Can you work these out from the model? Positions are in its coordinate system, mm. Round coordinates to 2 decimals unless told otherwise and drop trailing zeros. Order: outer loops, then holes, each group sorted by start corner. A loop starts at its lowest first (then second) coordinate and runs counter-clockwise, first axis right, second up.
Q1. If we section it at C-C (y = 50): Please give me the cut outline in (x, z).
Q2. If we section it at B-B (x = 0): Please give me the cut outline in (y, z), plus the area to 3 significant figures.
Q3. Will these pins go through, and if not, where does the flat tip stop? P1, Ø0.5, axis at x = 39.5, z = 1, coming from the -Y side; P2, Ø0.8, axis at y = 0.5, z = 0.5, coming from the -X side; P3, Ø0.5, axis at x = 52, z = 0.5, coming from the +Y side; P4, Ø0.5, axis at x = -40.5, z = 0.5, coming from the -Y side.
Q4. If we section it at A-A (y = 0): Please give me the cut outline in (x, z) (3 decimals), plus the area to 3 significant figures.
Q5. If we section it at D-D (z = 0.3): Count the separate pieces of the cut face and the enclosed holes in it, plus the area to 3 significant figures.
Q6. If I drill on line 1 (Y direction, x = 0, z = 0.55); line 2 (Y direction, x = 18.5, z = 1.45); line 3 (X direction, y = 46, z = 0.3) (3 decimals), over which ranges is the centre line in solid material (lowest first)?
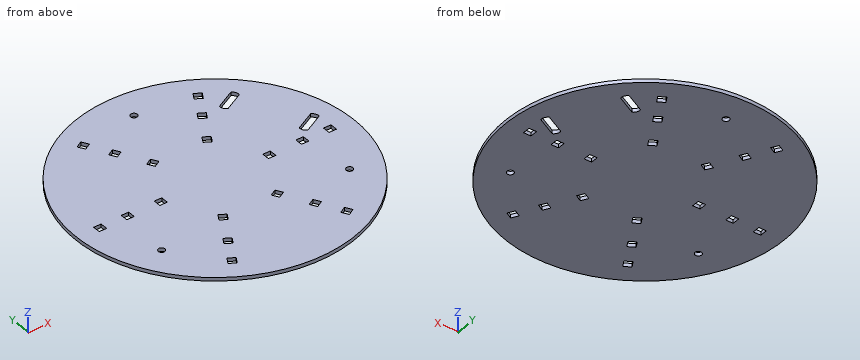
from build123d import *

# Parameters (mm, degrees)
SKETCH1_R           = 63.5
BOSS_EXTRUDE1_DEPTH = 1.6
SKETCH3_R           = 1.75
CUT_EXTRUDE4_DEPTH  = 1.6
SKETCH2_R           = 1.5
CUT_EXTRUDE5_DEPTH  = 1.6
CUT_EXTRUDE6_DEPTH  = 10
SKETCH5_W           = 3.45
SKETCH5_H           = 3.45
CUT_EXTRUDE7_DEPTH  = 10


with BuildPart() as part:
    # Sketch1 → Boss-Extrude1 (new body)
    with BuildSketch(Plane.XY):
        Circle(SKETCH1_R)
    extrude(amount=BOSS_EXTRUDE1_DEPTH)

    # Sketch3 → Cut-Extrude4 (cut)
    with BuildSketch(Plane(origin=(0, 0, 0), x_dir=(-1, 0, 0), z_dir=(0, 0, -1))):
        with Locations((-34.006305458, 36.654756705)):
            Circle(SKETCH3_R)
        with Locations((-49.354669589, 8.007283544)):
            Circle(SKETCH3_R)
    extrude(amount=-CUT_EXTRUDE4_DEPTH, mode=Mode.SUBTRACT)

    # Sketch2 → Cut-Extrude5 (cut)
    with BuildSketch(Plane(origin=(0, 0, 0), x_dir=(-1, 0, 0), z_dir=(0, 0, -1))):
        with Locations((0, 50)):
            Circle(SKETCH2_R)
        with Locations((43.301270189, -25)):
            Circle(SKETCH2_R)
        with Locations((-43.301270189, -25)):
            Circle(SKETCH2_R)
    extrude(amount=-CUT_EXTRUDE5_DEPTH, mode=Mode.SUBTRACT)

    # Sketch4 → Cut-Extrude6 (cut)
    with BuildSketch(Plane(origin=(0, 0, 0), x_dir=(-1, 0, 0), z_dir=(0, 0, -1))):
        with BuildLine():
            Line((-52.935522776, 11.911126581), (-44.12091565, 7.188553002))
            ThreePointArc((-44.12091565, 7.188553002), (-44.461118004, 5.385481223), (-45.773816402, 4.103440508))
            Line((-45.773816402, 4.103440508), (-54.588423529, 8.826014086))
            ThreePointArc((-54.588423529, 8.826014086), (-54.248221174, 10.629085865), (-52.935522776, 11.911126581))
        make_face()
        with BuildLine():
            Line((-39.240059397, 37.473487247), (-30.425452271, 32.750913668))
            ThreePointArc((-30.425452271, 32.750913668), (-29.112753873, 34.032954384), (-28.772551518, 35.836026163))
            Line((-28.772551518, 35.836026163), (-37.587158645, 40.558599742))
            ThreePointArc((-37.587158645, 40.558599742), (-38.899857043, 39.276559026), (-39.240059397, 37.473487247))
        make_face()
    extrude(amount=-CUT_EXTRUDE6_DEPTH, mode=Mode.SUBTRACT)

    # Sketch5 → Cut-Extrude7 (cut)
    with BuildSketch(Plane(origin=(0, 0, 0), x_dir=(-1, 0, 0), z_dir=(0, 0, -1))):
        with Locations((-52.94, 0)):
            Rectangle(SKETCH5_W, SKETCH5_H)
        Polygon((-24.113606178, -45.215991055), (-25.838606178, -48.203778698), (-28.826393822, -46.478778698), (-27.101393822, -43.490991055), align=None)
        Polygon((-27.101393822, 43.490991055), (-28.826393822, 46.478778698), (-25.838606178, 48.203778698), (-24.113606178, 45.215991055), align=None)
        with Locations((-40.24, 0)):
            Rectangle(SKETCH5_W, SKETCH5_H)
        with Locations((-25, 0)):
            Rectangle(SKETCH5_W, SKETCH5_H)
        with Locations((25, 0)):
            Rectangle(SKETCH5_W, SKETCH5_H)
        with Locations((40.24, 0)):
            Rectangle(SKETCH5_W, SKETCH5_H)
        with Locations((52.94, 0)):
            Rectangle(SKETCH5_W, SKETCH5_H)
        Polygon((13.131393822, -19.294241273), (14.856393822, -22.282028916), (11.868606178, -24.007028916), (10.143606178, -21.019241273), align=None)
        Polygon((20.751393822, -32.492468427), (22.476393822, -35.48025607), (19.488606178, -37.20525607), (17.763606178, -34.217468427), align=None)
        Polygon((24.113606178, -45.215991055), (25.838606178, -48.203778698), (28.826393822, -46.478778698), (27.101393822, -43.490991055), align=None)
        Polygon((-13.131393822, -19.294241273), (-14.856393822, -22.282028916), (-11.868606178, -24.007028916), (-10.143606178, -21.019241273), align=None)
        Polygon((-20.751393822, -32.492468427), (-22.476393822, -35.48025607), (-19.488606178, -37.20525607), (-17.763606178, -34.217468427), align=None)
        Polygon((-17.763606178, 34.217468427), (-19.488606178, 37.20525607), (-22.476393822, 35.48025607), (-20.751393822, 32.492468427), align=None)
        Polygon((-13.131393822, 19.294241273), (-14.856393822, 22.282028916), (-11.868606178, 24.007028916), (-10.143606178, 21.019241273), align=None)
        Polygon((10.143606178, 21.019241273), (11.868606178, 24.007028916), (14.856393822, 22.282028916), (13.131393822, 19.294241273), align=None)
        Polygon((17.763606178, 34.217468427), (19.488606178, 37.20525607), (22.476393822, 35.48025607), (20.751393822, 32.492468427), align=None)
        Polygon((24.113606178, 45.215991055), (25.838606178, 48.203778698), (28.826393822, 46.478778698), (27.101393822, 43.490991055), align=None)
    extrude(amount=-CUT_EXTRUDE7_DEPTH, mode=Mode.SUBTRACT)


solid = part.part
Solution:
1. outline: (-39.14, 0) - (-1.5, 0) - (-1.5, 1.6) - (-39.14, 1.6) - close; (1.5, 0) - (39.14, 0) - (39.14, 1.6) - (1.5, 1.6) - close
2. outline: (-63.5, 0) - (48.5, 0) - (48.5, 1.6) - (-63.5, 1.6) - close; (51.5, 0) - (63.5, 0) - (63.5, 1.6) - (51.5, 1.6) - close
2. area: 198 mm2
3. P1: stops at y = -49.92
3. P2: stops at x = -63.5
3. P3: stops at y = 36.8
3. P4: stops at y = -49.11
4. outline: (-63.5, 0) - (-54.665, 0) - (-54.665, 1.6) - (-63.5, 1.6) - close; (-51.215, 0) - (-41.965, 0) - (-41.965, 1.6) - (-51.215, 1.6) - close; (-38.515, 0) - (-26.725, 0) - (-26.725, 1.6) - (-38.515, 1.6) - close; (-23.275, 0) - (23.275, 0) - (23.275, 1.6) - (-23.275, 1.6) - close; (26.725, 0) - (38.515, 0) - (38.515, 1.6) - (26.725, 1.6) - close; (41.965, 0) - (51.215, 0) - (51.215, 1.6) - (41.965, 1.6) - close; (54.665, 0) - (63.5, 0) - (63.5, 1.6) - (54.665, 1.6) - close
4. area: 170 mm2
5. separate pieces: 1
5. enclosed holes: 23
5. area: 12,400 mm2
6. line 1: y = -63.5 to 48.5, 51.5 to 63.5
6. line 2: y = -60.75 to -35.49, -33.79 to 33.79, 35.49 to 60.75
6. line 3: x = -43.775 to -28.55, -24.566 to 24.566, 28.55 to 43.775
